Source: CAD feature listing. Evaluate the final solid. Frame: model axes, mm. Face numbers are marked on the shaded views. A direction names the side the tool comes from. Round coordinates to 2 decimals unless told otherwise and drop trailing zeros. Order: outer loops, then holes, each group sorted by start corner. A loop starts at its lowest first (then second) coordinate and runs counter-clockwise, first axis right, second up. Notation, with made-up numbers: (76, 67) - (119, 67) arc R9 ccw to (119, 72) - close; hole circle Ø1 at (62, 75.25). An arc over 180 degrees is marked (long way). Return JSON: item names as keys, results as strings. Group by question number.
1) Ray query, line 1 (Z direction, x = -3.75, y = 9.5); line 2 (Z direction, x = -7, y = -5); line 3 (Z direction, x = 1.5, y = 3.5). Return the intervals inside material, ascending. Write a range as from..to.
2) Access query for the marked faces 1 and 2. Directions: +Z, -Z, +X, -X, +Y, -Y. A direction counts if a zero-diameter tool reaches every point of the face in a straight line with its end or side. Return the directions, or none.
3) Section D-D, the plane z = 16.5. Return loops of the section in (x, y), plus the area to 3 significant figures.
4) Contact query for flat-ended pins moving along their axis: P1, Ø1.5, axis at x = -3, z = 23.5, coming from the +Y side; P2, Ø1, axis at x = -7, z = 16.5, coming from the +Y side; P3, Ø6, axis at x = 7, z = 26.5, coming from the +Y side; P4, Ø6, axis at x = 0.5, y = 7.5, coming from the +Z side. Output: stop coordinate, or through.
5) Section C-C, the plane z = 21. Return loops of the section in (x, y), plus the area to 3 significant figures.
6) Section A-A, the plane x = 0. Return loops of the section in (y, z), plus the area to 3 significant figures.
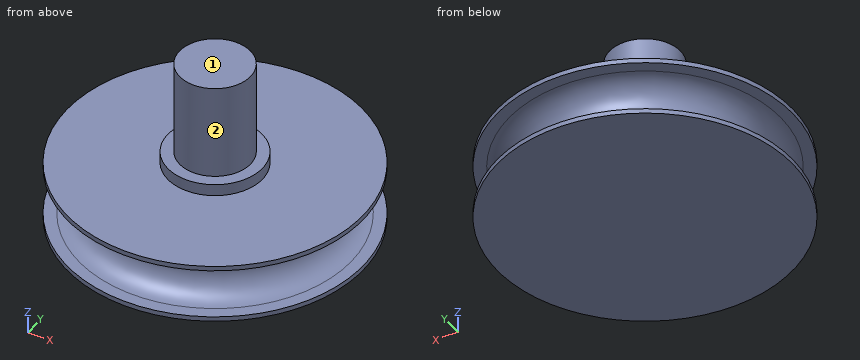
Solid Edge part; units mm, degrees
sketch "Sketch1" plane through (0, 0, 0) normal (0, -1, 0) x (1, 0, 0)
  line L0 (0, 18.72) -> (0, 13.72)
  line L1 (0, 13.72) -> (-11.5, 13.72)
  line L2 (-12.5, 13.72) -> (-11.5, 13.72)
  line L3 (-12.5, 14.12) -> (-12.5, 13.72)
  line L4 (-11.5, 14.12) -> (-12.5, 14.12)
  arc A0 (-11.5, 18.32) -> (-11.5, 14.12) centre (-11.5, 16.22) cw
  line L5 (-12.5, 18.32) -> (-11.5, 18.32)
  line L6 (-12.5, 18.72) -> (-12.5, 18.32)
  line L7 (-11.5, 18.72) -> (-12.5, 18.72)
  line L8 (-11.5, 18.72) -> (0, 18.72)
revolve "RevolvedProtrusion1" add sketch "Sketch1" angle 360 about axis through (0, 0, 54) along (0, 0, -1)
sketch "Sketch2" plane through (0, 0, 0) normal (0, -1, 0) x (1, 0, 0)
  line L0 (0, 18.72) -> (0, 27.72)
  line L1 (0, 27.72) -> (-3, 27.72)
  line L2 (-3, 27.72) -> (-3, 19.72)
  line L3 (-3, 19.72) -> (-4, 19.72)
  line L4 (-4, 19.72) -> (-4, 18.72)
  line L5 (-4, 18.72) -> (0, 18.72)
revolve "RevolvedProtrusion2" add sketch "Sketch2" angle 360 about axis through (0, 0, 54) along (0, 0, -1)
Geometry check:
{
 "1": {"line 1": "13.72..14.56, 17.88..18.72", "line 2": "13.72..18.72", "line 3": "13.72..19.72"},
 "2": {"face 1": "+Z, +X, -X, +Y, -Y", "face 2": "+Z"},
 "3": {"outline": "circle Ø18.84 at (0, 0)", "area": "279 mm2"},
 "4": {"P1": "y = 1.98", "P2": "y = 6.83", "P3": "through", "P4": "z = 18.72"},
 "5": {"outline": "circle Ø6 at (0, 0)", "area": "28.3 mm2"},
 "6": {"outline": "(-12.5, 13.72) - (12.5, 13.72) - (12.5, 14.12) - (11.5, 14.12) arc R2.1 cw to (11.5, 18.32) - (12.5, 18.32) - (12.5, 18.72) - (4, 18.72) - (4, 19.72) - (3, 19.72) - (3, 27.72) - (-3, 27.72) - (-3, 19.72) - (-4, 19.72) - (-4, 18.72) - (-12.5, 18.72) - (-12.5, 18.32) - (-11.5, 18.32) arc R2.1 cw to (-11.5, 14.12) - (-12.5, 14.12) - close", "area": "159 mm2"}
}
